Source: CAD feature listing. Evaluate the final solid. Frame: model axes, mm. A direction names the side the tool comes from. Give positions to 0.01 mm unless a question says otherwise; leave off trailing zeros. Order: outer loops, then holes, each group sorted by start corner. A loop starts at its lowest first (then second) coordinate and runs counter-clockwise, first axis right, second up. Notation, with made-up numbers: (-9.75, 52.5) - (31.25, 52.5) arc R17 cw to (31.25, 60.5) - close; hole circle Ø11 at (48, -24.75). An arc over 180 degrees is marked (long way). Answer as CSV lines item,"result".
```python
from build123d import *

# Parameters (mm, degrees)
SKETCH1_W           = 26.67
SKETCH1_H           = 52.07
BOSS_EXTRUDE1_DEPTH = 12.7
SKETCH2_W           = 21.59
SKETCH2_H           = 46.99
CUT_EXTRUDE1_DEPTH  = 10.16
BOSS_EXTRUDE2_REACH = 54.07


with BuildPart() as part:
    # Sketch1 → Boss-Extrude1 (new body)
    with BuildSketch(Plane(origin=(0, 0, 0), x_dir=(1, 0, 0), z_dir=(0, 1, 0))):
        with Locations((13.335, 26.035)):
            Rectangle(SKETCH1_W, SKETCH1_H)
    extrude(amount=BOSS_EXTRUDE1_DEPTH)

    # Sketch2 → Cut-Extrude1 (cut)
    with BuildSketch(Plane(origin=(0, 12.7, 0), x_dir=(1, 0, 0), z_dir=(0, 1, 0))):
        with Locations((13.335, 26.035)):
            Rectangle(SKETCH2_W, SKETCH2_H)
    extrude(amount=-CUT_EXTRUDE1_DEPTH, mode=Mode.SUBTRACT)

    # Sketch4 → Boss-Extrude2 (add, up to next)
    with BuildSketch(Plane.XY, mode=Mode.PRIVATE) as boss_extrude2_sk1:
        with BuildLine():
            Line((8.89, 0), (17.78, 0))
            ThreePointArc((17.78, 0), (14.953468796, 1.200296929), (13.335, 3.81))
            ThreePointArc((13.335, 3.81), (11.716531204, 1.200296929), (8.89, 0))
        make_face()
    boss_extrude2_tool1 = extrude(boss_extrude2_sk1.sketch, amount=-BOSS_EXTRUDE2_REACH, mode=Mode.PRIVATE) - part.part
    add(boss_extrude2_tool1.solids().sort_by_distance((13.335, 0.99851, 0))[0])


solid = part.part
```
(1) Cut plane A-A (y = 9.5). Return loops of the section in (x, z).
Completed:
outline,"(0, -52.07) - (26.67, -52.07) - (26.67, 0) - (0, 0) - close; hole (2.54, -49.53) - (24.13, -49.53) - (24.13, -2.54) - (2.54, -2.54) - close"
(2) Ray query, line 1 (X direction, y = 8, z = -6.5); line 2 (Z direction, x = 15.25, y = 5); line 3 (Y direction, x = 12.5, z = -28.5). Return the intervals inside material, ascending. Write a range as from..to.
Completed:
line 1,"0..2.54, 24.13..26.67"
line 2,"-52.07..-49.53, -2.54..0"
line 3,"0..2.54"
(3) Access query for faces 1 (the flat face through (24.13, 8, -26)), 2 (the flat face through (0, 6, -26)). Directions: +Z, -Z, +X, -X, +Y, -Y. A direction counts if a zero-diameter tool reaches every point of the face in a straight line with its end or side. Return the directions, or none.
Completed:
face 1,"+Y"
face 2,"+Z, -Z, -X, +Y, -Y"
(4) Mould query, pull axis X, two halves, no side actions, for faces 3 (the flat face through (13, 6, -52.07)), 4 (the cylindrical face through (13.126, 3.167, -25.706)), 5 (the flat face through (26.67, 6, -26)). Classes: released by +X, released by -X, zero draft, split by the parting line, or undercut.
Completed:
face 3,"zero draft"
face 4,"undercut"
face 5,"released by +X"
(5) Contact query for flat-ended pins moving along their axis: pin 1 (10 mm diameter, centred on x = 19, z = -41, fed in from -Y); pin 2 (3 mm diameter, centred on x = 8, z = -17.5, fed in from +Y). Output: stop coordinate, or through.
Completed:
pin 1,"y = 0"
pin 2,"y = 2.54"
(6) Cut plane C-C (z = -17). Return loops of the section in (x, y) (3 decimals), then the cut area to 3 significant figures.
Completed:
outline,"(0, 0) - (26.67, 0) - (26.67, 12.7) - (24.13, 12.7) - (24.13, 2.54) - (13.847, 2.54) arc R5.08 cw to (13.335, 3.81) arc R5.08 cw to (12.823, 2.54) - (2.54, 2.54) - (2.54, 12.7) - (0, 12.7) - close"
area,"120 mm²"
(7) Cut plane B-B (x = 5.5). Return loops of the section in (y, z).
Completed:
outline,"(0, -52.07) - (12.7, -52.07) - (12.7, -49.53) - (2.54, -49.53) - (2.54, -2.54) - (12.7, -2.54) - (12.7, 0) - (0, 0) - close"
